Read the model definition and answer for the solid it produces. Units are mm, in the model's axes. A direction names the side the tool comes from. Round coordinates to 2 decimals unless told otherwise and drop trailing zeros. Write each loop counter-clockwise with the first axis right and the second up, starting at its lowest first coordinate (ties: lowest second). Pieces come first, ordered by that corner, then holes. Notation, with made-up numbers: (14, -26) -> (22, -26) arc R19 cw to (22, 4) -> close; hole circle Ø5 at (37.5, -25). An arc over 180 degrees is marked (long way). Return JSON: item names as keys, results as strings. Group by question number.
(1) For faces 4 (the cylindrical face through (-5.29, -8.57, 3.04)), 5 (the cylindrical face through (2.384, 9.787, 3.042)), 6 (the cylindrical face through (-3.826, -9.288, 3.042)), determine the directions among +Z, -Z, +X, -X, +Y, -Y from which every point of the face is accessible in a straight line to the end or side of a thin tool.
(2) Straight lines are drawn through the part: line 1 (X direction, y = 0, z = 2.5); line 2 (Y direction, x = 0, z = 4.25); line 3 (Y direction, x = -8.25, z = 1.25). For each, find the intervals that lie inside material, in ascending order.
(3) A cutting plane is placed at B-B on y = 5.75. Give the vertices of the cut face in (x, z), then the cut area to 3 significant figures.
(4) A cutting plane is placed at A-A on y = 9.75. Give the vertices of the cut face in (x, z).
(5) The mould has two halves that part along Y. Classify faces 1 (the cylindrical face through (0.76, -10.04, 3.04)), 2 (the cylindrical face through (3.826, 9.288, 3.042)), 3 (the cylindrical face through (5.29, 8.57, 3.04)): released by +Y, released by -Y, zero draft, split by the parting line, or undercut.
(6) Given pin 1 (2 mm diameter, centred on y = 2.5, z = 2.5, fed in from +X), flat-ended and moving along its own axis, determine where the tip first touches the part or whether it passes through.
```python
from build123d import *

# Parameters (mm, degrees)
CUT_EXTRUDE1_DEPTH  = 20.646882704
CIRPATTERN1_COUNT   = 20
SKETCH5_R           = 7.15
SKETCH5_R_2         = 2
BOSS_EXTRUDE1_DEPTH = 6
CUT_EXTRUDE2_REACH  = 18.673
SKETCH6_R           = 5.85
BOSS_EXTRUDE2_DEPTH = 3


with BuildPart() as part:
    # Sketch3 → Revolve1 (revolve)
    with BuildSketch(Plane(origin=(0, 0, 0), x_dir=(0, 0, -1), z_dir=(1, 0, 0)), mode=Mode.PRIVATE) as revolve1_sk:
        Polygon((-6, 11), (0, 11), (0, 7.15), (-1.714285714, 7.15), (-1.714285714, 5.85), (6, 5.85), (6, 2.5), (-6, 2.5), (-6, 5.85), (-4.285714286, 5.85), (-4.285714286, 7.15), (-6, 7.15), align=None)
    revolve(revolve1_sk.sketch.rotate(Axis((0, 0, -6), (0, 0, 1)), 90), axis=Axis((0, 0, -6), (0, 0, 1)))

    # Sketch4 → Cut-Extrude1 (cut, symmetric)
    with BuildSketch(Plane.XY.offset(6)):
        with BuildLine():
            ThreePointArc((-0.206650348, 10.998058721), (-0.762582532, 10.030093075), (-0.998187985, 8.938988976))
            ThreePointArc((-0.998187985, 8.938988976), (-1.076668536, 8.753613059), (-1.254660723, 8.65958004))
            ThreePointArc((-1.254660723, 8.65958004), (-1.368801569, 8.64227298), (-1.48270414, 8.623461511))
            ThreePointArc((-1.48270414, 8.623461511), (-1.681042571, 8.657889616), (-1.812966318, 8.809940765))
            ThreePointArc((-1.812966318, 8.809940765), (-2.374210129, 9.77483634), (-3.20205089, 10.523633883))
            ThreePointArc((-3.20205089, 10.523633883), (-1.720779115, 10.864571747), (-0.206650348, 10.998058721))
        make_face()
    cut_extrude1 = extrude(amount=CUT_EXTRUDE1_DEPTH, both=True, mode=Mode.SUBTRACT)

    # CirPattern1: Cut-Extrude1 ×20 about axis
    cirpattern1_axis = Axis((0, 0, 0), (0, 0, 1))
    for i in range(1, CIRPATTERN1_COUNT):
        add(cut_extrude1.rotate(cirpattern1_axis, i * 360 / CIRPATTERN1_COUNT), mode=Mode.SUBTRACT)

    # Sketch5 → Boss-Extrude1 (add)
    with BuildSketch(Plane.XY.offset(6)):
        Circle(SKETCH5_R)
        Circle(SKETCH5_R_2, mode=Mode.SUBTRACT)
    extrude(amount=-BOSS_EXTRUDE1_DEPTH)

    # Sketch6 → Cut-Extrude2 (cut, up to next)
    with BuildSketch(Plane(origin=(0, 0, 0), x_dir=(-1, 0, 0), z_dir=(0, 0, -1)), mode=Mode.PRIVATE) as cut_extrude2_sk1:
        Circle(SKETCH6_R)
    cut_extrude2_tool1 = extrude(cut_extrude2_sk1.sketch, amount=CUT_EXTRUDE2_REACH, mode=Mode.PRIVATE) & part.part
    add(cut_extrude2_tool1.solids().sort_by_distance((0, 0, 0))[0], mode=Mode.SUBTRACT)

    # 3DSketch1 → Boss-Extrude2 (add)
    with BuildSketch(Plane(origin=(-1.5, -1.322875656, 6), x_dir=(0.4472135954999579, 0, -0.894427190999916), z_dir=(0, -1, 0))):
        Polygon((0, 0), (1.341640786, 2.683281573), (6.708203932, 0), (5.366563146, -2.683281573), align=None)
    extrude(amount=BOSS_EXTRUDE2_DEPTH)


solid = part.part
```
Checks:
{
 "1": {"face 4": "+Z, -Z, -Y", "face 5": "+Z, -Z, +Y", "face 6": "+Z, -Z"},
 "2": {"line 1": "x = -11 to -2, 2 to 11", "line 2": "y = -11 to -1.32, 2 to 11", "line 3": "y = -6.62 to -4.86, -3.73 to 3.73, 4.86 to 6.62"},
 "3": {"outline": "(-8.82, 0) -> (8.82, 0) -> (8.82, 6) -> (-8.82, 6) -> close", "area": "106 mm^2"},
 "4": {"outline": "(-3.77, 0) -> (-2.35, 0) -> (-2.35, 6) -> (-3.77, 6) -> close; (-0.86, 0) -> (0.86, 0) -> (0.86, 6) -> (-0.86, 6) -> close; (2.35, 0) -> (3.77, 0) -> (3.77, 6) -> (2.35, 6) -> close"},
 "5": {"face 1": "released by -Y", "face 2": "undercut", "face 3": "released by +Y"},
 "6": {"pin 1": "stops at x = 10.52"}
}
